from build123d import *

# Parameters (mm, degrees)
SKETCH1_W                      = 1155
SKETCH1_H                      = 55
BASE_FLANGE1_DEPTH             = 2.5
EDGE_FLANGE1_STRIP_W           = 11.4732
EDGE_FLANGE1_STRIP_H           = 2.5
EDGE_FLANGE1_STRIP_CUT_DEPTH   = 1155
EDGE_FLANGE1_STRIP_2_W         = 11.4732
EDGE_FLANGE1_STRIP_2_H         = 2.5
EDGE_FLANGE1_STRIP_CUT_2_DEPTH = 1155
EDGE_FLANGE1_DEPTH             = 1155
EDGE_FLANGE1_BEND_DEPTH        = 1155
CUT_EXTRUDE1_DEPTH             = 581.673316074
CUT_EXTRUDE1_DEPTH_BACK        = 581.673316074
SKETCH13_R                     = 6
CUT_EXTRUDE2_DEPTH             = 581.673316074
LPATTERN1_COUNT                = 2
LPATTERN1_PITCH                = 70
SKETCH14_R                     = 4.5
CUT_EXTRUDE3_DEPTH             = 10


# Sheet-metal steps are written as plain solids
with BuildPart() as part:
    # Sketch1 → Base-Flange1 (new body)
    with BuildSketch(Plane.XY):
        Rectangle(SKETCH1_W, SKETCH1_H)
    extrude(amount=-BASE_FLANGE1_DEPTH)

    # Edge-Flange1 strip (across the edge) → Edge-Flange1 strip cut (cut)
    with BuildSketch(Plane(origin=(577.5, 27.5, 0), x_dir=(0, -1, 0), z_dir=(-1, 0, 0))):
        with Locations((-2.5, -1.25)):
            Rectangle(EDGE_FLANGE1_STRIP_W, EDGE_FLANGE1_STRIP_H)
    extrude(amount=EDGE_FLANGE1_STRIP_CUT_DEPTH, mode=Mode.SUBTRACT)

    # Edge-Flange1 strip 2 (across the edge) → Edge-Flange1 strip cut 2 (cut)
    with BuildSketch(Plane(origin=(-577.5, -27.5, 0), x_dir=(0, 1, 0), z_dir=(1, 0, 0))):
        with Locations((-2.5, -1.25)):
            Rectangle(EDGE_FLANGE1_STRIP_2_W, EDGE_FLANGE1_STRIP_2_H)
    extrude(amount=EDGE_FLANGE1_STRIP_CUT_2_DEPTH, mode=Mode.SUBTRACT)

    # Edge-Flange1 section (across the edge) → Edge-Flange1 (add)
    with BuildSketch(Plane(origin=(577.5, 27.5, 0), x_dir=(0, -1, 0), z_dir=(-1, 0, 0))):
        with BuildLine():
            Line((0, 0.7366), (0, 25.5))
            Line((0, 25.5), (2.5, 25.5))
            Line((2.5, 25.5), (2.5, 0.7366))
            ThreePointArc((2.5, 0.7366), (2.715745145, 0.215745145), (3.2366, 0))
            Line((3.2366, 0), (3.2366, -2.5))
            ThreePointArc((3.2366, -2.5), (0.947978192, -1.552021808), (0, 0.7366))
        make_face()
    extrude(amount=EDGE_FLANGE1_DEPTH)

    # Edge-Flange1 section 2 (across the edge) → Edge-Flange1 bend (add)
    with BuildSketch(Plane(origin=(-577.5, -27.5, 0), x_dir=(0, 1, 0), z_dir=(1, 0, 0))):
        with BuildLine():
            Line((0, 0.7366), (0, 25.5))
            Line((0, 25.5), (2.5, 25.5))
            Line((2.5, 25.5), (2.5, 0.7366))
            ThreePointArc((2.5, 0.7366), (2.715745145, 0.215745145), (3.2366, 0))
            Line((3.2366, 0), (3.2366, -2.5))
            ThreePointArc((3.2366, -2.5), (0.947978192, -1.552021808), (0, 0.7366))
        make_face()
    extrude(amount=EDGE_FLANGE1_BEND_DEPTH)

    # Sketch12 → Cut-Extrude1 (cut, two sides: drawn at the far end of the back side and taken through both)
    with BuildSketch(Plane(origin=(0, 27.5, 0), x_dir=(1, 0, 0), z_dir=(0, 1, 0)).offset(-CUT_EXTRUDE1_DEPTH_BACK)):
        with BuildLine():
            Line((572.5, -17), (558.5, -17))
            ThreePointArc((558.5, -17), (555.5, -14), (558.5, -11))
            Line((558.5, -11), (572.5, -11))
            ThreePointArc((572.5, -11), (575.5, -14), (572.5, -17))
        make_face()
    extrude(amount=CUT_EXTRUDE1_DEPTH + CUT_EXTRUDE1_DEPTH_BACK, mode=Mode.SUBTRACT)

    # Sketch13 → Cut-Extrude2 (cut, symmetric)
    with BuildSketch(Plane(origin=(0, 27.5, 0), x_dir=(1, 0, 0), z_dir=(0, 1, 0))):
        with Locations(Location((-554.5, -14, 0), (0, 0, 270))):
            Circle(SKETCH13_R)
    cut_extrude2 = extrude(amount=CUT_EXTRUDE2_DEPTH, both=True, mode=Mode.SUBTRACT)

    # LPattern1: Cut-Extrude2 ×2
    with Locations(*[(i * LPATTERN1_PITCH, 0, 0) for i in range(1, LPATTERN1_COUNT)]):
        add(cut_extrude2, mode=Mode.SUBTRACT)

    # Sketch14 → Cut-Extrude3 (cut)
    with BuildSketch(Plane.XY):
        with Locations((44.9385, 0)):
            Circle(SKETCH14_R)
    extrude(amount=-CUT_EXTRUDE3_DEPTH, mode=Mode.SUBTRACT)


solid = part.part
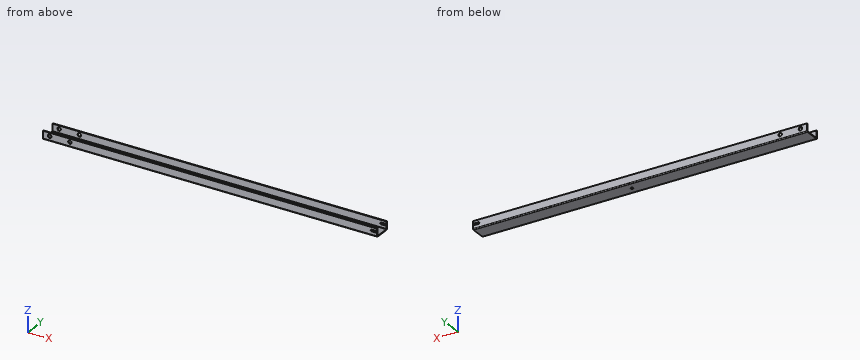
Geometry: final body of the model. Coordinates: model frame, mm. Coordinates: 2 decimals unless noted, no trailing zeros. Order: outer loops, then holes, each group sorted by start corner. A loop starts at its lowest first (then second) coordinate and runs counter-clockwise, first axis right, second up.
(1) Section query A-A (x = -337). Return the cut outline in (y, z).
(2) Section query B-B (y = -15.5). Return the cut outline in (x, z), plus the area to 3 significant figures.
(3) Material intervals for probe 1 along X at (y, z) = (-26.6, 14); probe 2 along Y at (x, z) = (-97, 18); probe 3 along Z at (x, y) = (258.5, 13.5), sorted ascending.
(4) First-contact query: pin 1 (0.8 mm diameter, centred on x = 567, y = 26, fed in from -Z); pin 2 (6 mm diameter, centred on x = -94, y = 13.5, fed in from +Z); pin 3 (14 mm diameter, centred on x = -484.5, z = 14, fed in from -Y); pin 4 (2 mm diameter, centred on x = 566.5, y = -25.5, fed in from -Z). Flat tips, straight axial feed; report the tip coordinate or a pass-through.
Solution:
1. outline: (-27.5, 0.74) arc R3.24 ccw to (-24.26, -2.5) - (24.26, -2.5) arc R3.24 ccw to (27.5, 0.74) - (27.5, 25.5) - (25, 25.5) - (25, 0.74) arc R0.74 cw to (24.26, 0) - (-24.26, 0) arc R0.74 cw to (-25, 0.74) - (-25, 25.5) - (-27.5, 25.5) - close
2. outline: (-577.5, -2.5) - (577.5, -2.5) - (577.5, 0) - (-577.5, 0) - close
2. area: 2,890 mm2
3. probe 1: x = -577.5 to -560.5, -548.5 to -490.5, -478.5 to 555.5, 575.5 to 577.5
3. probe 2: y = -27.5 to -25, 25 to 27.5
3. probe 3: z = -2.5 to 0
4. pin 1: stops at z = -2.21
4. pin 2: stops at z = 0
4. pin 3: stops at y = -27.5
4. pin 4: stops at z = -2.49
